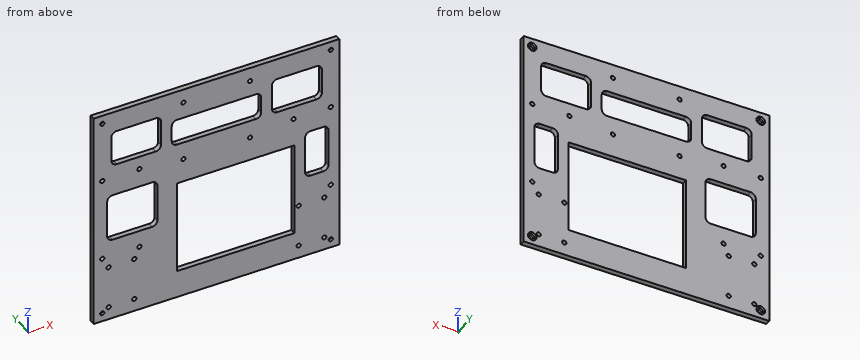
```python
from build123d import *

# Parameters (mm, degrees)
SKETCH1_W           = 119
SKETCH1_H           = 103
BOSS_EXTRUDE1_DEPTH = 2.5
SKETCH3_W           = 55
SKETCH3_H           = 44
CUT_EXTRUDE2_DEPTH  = 10
SKETCH4_W           = 103
SKETCH4_H           = 2.5
BOSS_EXTRUDE2_DEPTH = 1.5
SKETCH5_W           = 103
SKETCH5_H           = 2.5
BOSS_EXTRUDE3_DEPTH = 1.5
SKETCH6_W           = 103
SKETCH6_H           = 2.5
CUT_EXTRUDE3_DEPTH  = 3.5
SKETCH7_W           = 103
SKETCH7_H           = 2.5
CUT_EXTRUDE4_DEPTH  = 3.5
SKETCH8_R           = 1
CUT_EXTRUDE5_DEPTH  = 10
SKETCH9_R           = 1
CUT_EXTRUDE6_DEPTH  = 10
SKETCH10_R          = 2
CUT_EXTRUDE7_DEPTH  = 1.25
SKETCH11_R          = 1
CUT_EXTRUDE8_DEPTH  = 11
CUT_EXTRUDE9_DEPTH  = 11


with BuildPart() as part:
    # Sketch1 → Boss-Extrude1 (new body)
    with BuildSketch(Plane(origin=(0, 0, 0), x_dir=(1, 0, 0), z_dir=(0, 1, 0))):
        Rectangle(SKETCH1_W, SKETCH1_H)
    extrude(amount=BOSS_EXTRUDE1_DEPTH)

    # Sketch3 → Cut-Extrude2 (cut)
    with BuildSketch(Plane(origin=(0, 2.5, 0), x_dir=(1, 0, 0), z_dir=(0, 1, 0))):
        with Locations((9, 16.5)):
            Rectangle(SKETCH3_W, SKETCH3_H)
    extrude(amount=-CUT_EXTRUDE2_DEPTH, mode=Mode.SUBTRACT)

    # Sketch4 → Boss-Extrude2 (add)
    with BuildSketch(Plane.ZY.offset(59.5)):
        with Locations((0, 1.25)):
            Rectangle(SKETCH4_W, SKETCH4_H)
    extrude(amount=BOSS_EXTRUDE2_DEPTH)

    # Sketch5 → Boss-Extrude3 (add)
    with BuildSketch(Plane(origin=(59.5, 0, 0), x_dir=(0, 0, -1), z_dir=(1, 0, 0))):
        with Locations((0, 1.25)):
            Rectangle(SKETCH5_W, SKETCH5_H)
    extrude(amount=BOSS_EXTRUDE3_DEPTH)

    # Sketch6 → Cut-Extrude3 (cut)
    with BuildSketch(Plane.ZY.offset(61)):
        with Locations((0, 1.25)):
            Rectangle(SKETCH6_W, SKETCH6_H)
    extrude(amount=-CUT_EXTRUDE3_DEPTH, mode=Mode.SUBTRACT)

    # Sketch7 → Cut-Extrude4 (cut)
    with BuildSketch(Plane(origin=(61, 0, 0), x_dir=(0, 0, -1), z_dir=(1, 0, 0))):
        with Locations((0, 1.25)):
            Rectangle(SKETCH7_W, SKETCH7_H)
    extrude(amount=-CUT_EXTRUDE4_DEPTH, mode=Mode.SUBTRACT)

    # Sketch8 → Cut-Extrude5 (cut)
    with BuildSketch(Plane(origin=(0, 2.5, 0), x_dir=(1, 0, 0), z_dir=(0, 1, 0))):
        with Locations((-15.5, -44.96)):
            Circle(SKETCH8_R)
        with Locations((15.7, -44.96)):
            Circle(SKETCH8_R)
        with Locations((-15.5, -16.63)):
            Circle(SKETCH8_R)
        with Locations((15.7, -16.63)):
            Circle(SKETCH8_R)
        with Locations((-53.5, -18.81)):
            Circle(SKETCH8_R)
        with Locations((-36.1, -18.81)):
            Circle(SKETCH8_R)
        with Locations((-53.5, 20.19)):
            Circle(SKETCH8_R)
        with Locations((-36.1, 20.19)):
            Circle(SKETCH8_R)
        with Locations((36.1, -18.81)):
            Circle(SKETCH8_R)
        with Locations((53.5, -18.81)):
            Circle(SKETCH8_R)
        with Locations((53.5, 20.19)):
            Circle(SKETCH8_R)
    extrude(amount=-CUT_EXTRUDE5_DEPTH, mode=Mode.SUBTRACT)

    # Sketch9 → Cut-Extrude6 (cut)
    with BuildSketch(Plane(origin=(0, 2.5, 0), x_dir=(1, 0, 0), z_dir=(0, 1, 0))):
        with Locations((-53.5, 47.5)):
            Circle(SKETCH9_R)
        with Locations((53.5, -47.5)):
            Circle(SKETCH9_R)
        with Locations((53.5, 47.5)):
            Circle(SKETCH9_R)
        with Locations((-53.5, -47.5)):
            Circle(SKETCH9_R)
    extrude(amount=-CUT_EXTRUDE6_DEPTH, mode=Mode.SUBTRACT)

    # Sketch10 → Cut-Extrude7 (cut)
    with BuildSketch(Plane(origin=(0, 2.5, 0), x_dir=(1, 0, 0), z_dir=(0, 1, 0))):
        with Locations((-53.5, 47.5)):
            Circle(SKETCH10_R)
        with Locations((-53.5, -47.5)):
            Circle(SKETCH10_R)
        with Locations((53.5, -47.5)):
            Circle(SKETCH10_R)
        with Locations((53.5, 47.5)):
            Circle(SKETCH10_R)
    extrude(amount=-CUT_EXTRUDE7_DEPTH, mode=Mode.SUBTRACT)

    # Sketch11 → Cut-Extrude8 (cut)
    with BuildSketch(Plane(origin=(0, 2.5, 0), x_dir=(1, 0, 0), z_dir=(0, 1, 0))):
        with Locations((-50.5, 45.5)):
            Circle(SKETCH11_R)
        with Locations((-50.5, 25.5)):
            Circle(SKETCH11_R)
        with Locations((-38.5, 45.5)):
            Circle(SKETCH11_R)
        with Locations((-38.5, 25.5)):
            Circle(SKETCH11_R)
        with Locations((50.5, 25.5)):
            Circle(SKETCH11_R)
        with Locations((38.5, 25.5)):
            Circle(SKETCH11_R)
        with Locations((38.5, 45.5)):
            Circle(SKETCH11_R)
        with Locations((50.5, 45.5)):
            Circle(SKETCH11_R)
    extrude(amount=-CUT_EXTRUDE8_DEPTH, mode=Mode.SUBTRACT)

    # Sketch12 → Cut-Extrude9 (cut)
    with BuildSketch(Plane(origin=(0, 2.5, 0), x_dir=(1, 0, 0), z_dir=(0, 1, 0))):
        with BuildLine():
            Line((-46.739053949, -24.945491093), (-28.457129996, -24.945491093))
            ThreePointArc((-28.457129996, -24.945491093), (-26.689363043, -25.67772414), (-25.957129996, -27.445491093))
            Line((-25.957129996, -27.445491093), (-25.957129996, -39.065269049))
            ThreePointArc((-25.957129996, -39.065269049), (-26.689363043, -40.833036002), (-28.457129996, -41.565269049))
            Line((-28.457129996, -41.565269049), (-46.739053949, -41.565269049))
            ThreePointArc((-46.739053949, -41.565269049), (-48.506820902, -40.833036002), (-49.239053949, -39.065269049))
            Line((-49.239053949, -39.065269049), (-49.239053949, -27.445491093))
            ThreePointArc((-49.239053949, -27.445491093), (-48.506820902, -25.67772414), (-46.739053949, -24.945491093))
        make_face()
        with BuildLine():
            Line((-48.675698452, -10.035902375), (-30.13630944, -10.035902375))
            ThreePointArc((-30.13630944, -10.035902375), (-28.368542487, -9.303669328), (-27.63630944, -7.535902375))
            Line((-27.63630944, -7.535902375), (-27.63630944, 9.759475357))
            ThreePointArc((-27.63630944, 9.759475357), (-28.368542487, 11.52724231), (-30.13630944, 12.259475357))
            Line((-30.13630944, 12.259475357), (-48.675698452, 12.259475357))
            ThreePointArc((-48.675698452, 12.259475357), (-50.443465405, 11.52724231), (-51.175698452, 9.759475357))
            Line((-51.175698452, 9.759475357), (-51.175698452, -7.535902375))
            ThreePointArc((-51.175698452, -7.535902375), (-50.443465405, -9.303669328), (-48.675698452, -10.035902375))
        make_face()
        with BuildLine():
            Line((-20.957129996, -27.445491093), (-20.957129996, -34.866758765))
            ThreePointArc((-20.957129996, -34.866758765), (-20.224896949, -36.634525718), (-18.457129996, -37.366758765))
            Line((-18.457129996, -37.366758765), (18.457129996, -37.366758765))
            ThreePointArc((18.457129996, -37.366758765), (20.224896949, -36.634525718), (20.957129996, -34.866758765))
            Line((20.957129996, -34.866758765), (20.957129996, -27.445491093))
            ThreePointArc((20.957129996, -27.445491093), (20.224896949, -25.67772414), (18.457129996, -24.945491093))
            Line((18.457129996, -24.945491093), (-18.457129996, -24.945491093))
            ThreePointArc((-18.457129996, -24.945491093), (-20.224896949, -25.67772414), (-20.957129996, -27.445491093))
        make_face()
        with BuildLine():
            Line((28.457129996, -41.565269049), (46.850265705, -41.565269049))
            ThreePointArc((46.850265705, -41.565269049), (48.618032658, -40.833036002), (49.350265705, -39.065269049))
            Line((49.350265705, -39.065269049), (49.350265705, -27.445491093))
            ThreePointArc((49.350265705, -27.445491093), (48.618032658, -25.67772414), (46.850265705, -24.945491093))
            Line((46.850265705, -24.945491093), (28.457129996, -24.945491093))
            ThreePointArc((28.457129996, -24.945491093), (26.689363043, -25.67772414), (25.957129996, -27.445491093))
            Line((25.957129996, -27.445491093), (25.957129996, -39.065269049))
            ThreePointArc((25.957129996, -39.065269049), (26.689363043, -40.833036002), (28.457129996, -41.565269049))
        make_face()
        with BuildLine():
            Line((41.5, 9.759475357), (41.5, -7.535902375))
            ThreePointArc((41.5, -7.535902375), (42.232233047, -9.303669328), (44, -10.035902375))
            Line((44, -10.035902375), (50, -10.035902375))
            ThreePointArc((50, -10.035902375), (51.767766953, -9.303669328), (52.5, -7.535902375))
            Line((52.5, -7.535902375), (52.5, 9.759475357))
            ThreePointArc((52.5, 9.759475357), (51.767766953, 11.52724231), (50, 12.259475357))
            Line((50, 12.259475357), (44, 12.259475357))
            ThreePointArc((44, 12.259475357), (42.232233047, 11.52724231), (41.5, 9.759475357))
        make_face()
    extrude(amount=-CUT_EXTRUDE9_DEPTH, mode=Mode.SUBTRACT)


solid = part.part
```
Model file for the job. Use its own axes, mm. Give positions to 0.01 mm unless a question says otherwise; leave off trailing zeros. Loops run counter-clockwise (first coordinate to the right, second up) from the corner with the lowest first, then second, coordinate; pieces in that order, holes last. Notation, with made-up numbers: (-23.75, -33) - (-1.75, -33) arc R18 cw to (-1.75, -21) - close; hole circle Ø7 at (-30, 42). An arc over 180 degrees is marked (long way). One line per item, written item: value. Start each with the question number.
1. Slice it at D-D (x = -33). List the corners of the cut face in (y, z).
2. Probe L1, parallel to Z at x = -9, y = 0.85; L2, parallel to X at y = 0.7, z = 18.81; L3, parallel to X at y = 1.8, z = 44.96. List the from-to ranges inside material, lowest first. Write a range as from..to.
3. Slice it at C-C (z = -37). List the corners of the cut face in (x, y).
4. Slice it at A-A (x = -6). List the corners of the cut face in (y, z).
5. Slice it at B-B (z = -3). List the corners of the cut face in (x, y).
6. Pin check, flat tips, straight feed: pin 1 (1.2 mm diameter, centred on x = -15.5, z = 16.63, fed in from +Y); pin 2 (2 mm diameter, centred on x = 54, z = 48, fed in from +Y). Stop position of each tip, or through.
Solution:
1. outline: (0, -51.5) - (2.5, -51.5) - (2.5, -12.26) - (0, -12.26) - close; (0, 10.04) - (2.5, 10.04) - (2.5, 24.95) - (0, 24.95) - close; (0, 41.57) - (2.5, 41.57) - (2.5, 51.5) - (0, 51.5) - close
2. L1: z = -51.5..-38.5, 5.5..24.95, 37.37..51.5
2. L2: x = -57.5..-54.5, -52.5..-37.1, -35.1..35.1, 37.1..52.5, 54.5..57.5
2. L3: x = -57.5..-16.5, -14.5..14.7, 16.7..57.5
3. outline: (-57.5, 0) - (-18.5, 0) - (-18.5, 2.5) - (-57.5, 2.5) - close; (36.5, 0) - (57.5, 0) - (57.5, 2.5) - (36.5, 2.5) - close
4. outline: (0, -51.5) - (2.5, -51.5) - (2.5, -38.5) - (0, -38.5) - close; (0, 5.5) - (2.5, 5.5) - (2.5, 24.95) - (0, 24.95) - close; (0, 37.37) - (2.5, 37.37) - (2.5, 51.5) - (0, 51.5) - close
5. outline: (-57.5, 0) - (-51.18, 0) - (-51.18, 2.5) - (-57.5, 2.5) - close; (-27.64, 0) - (-18.5, 0) - (-18.5, 2.5) - (-27.64, 2.5) - close; (36.5, 0) - (41.5, 0) - (41.5, 2.5) - (36.5, 2.5) - close; (52.5, 0) - (57.5, 0) - (57.5, 2.5) - (52.5, 2.5) - close
6. pin 1: passes through
6. pin 2: stops at y = 1.25
